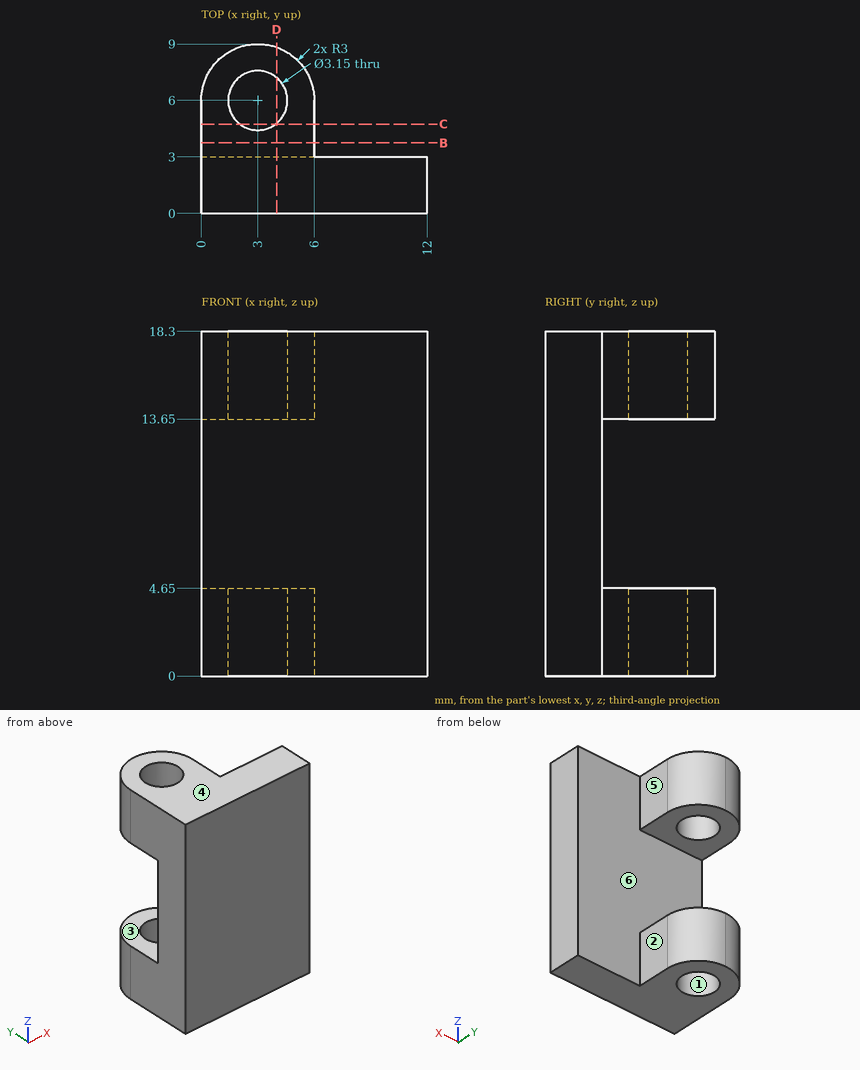
Job drawing, mm, ordinate dimensions from the low corner. One solid piece. A direction names the side the tool comes from. Round coordinates to 2 decimals unless told otherwise and drop trailing zeros. Order: outer loops, then holes, each group sorted by start corner. A loop starts at its lowest first (then second) coordinate and runs counter-clockwise, first axis right, second up. Notation, with made-up numbers: (84.25, 88) -> (138.25, 88) arc R22 cw to (138.25, 110) -> close; hole circle Ø1 at (-5.75, -17.75). An arc over 180 degrees is marked (long way). Write item = value, one per line.
(1) 3-axis set-ups, long thin cutter, end or side, ignore diameter. For the marked faces 1, 2 and 3: which of +Z, -Z, +X, -X, +Y, -Y reach the whole face in a straight line?
Answers follow:
face_1 = +Z, -Z
face_2 = +Z, -Z, +X, +Y
face_3 = +X, -X, +Y
(2) Cut at C-C (y = 4.75). Write the cut outline in (x, z).
Answers follow:
outline = (0, 0) -> (2.04, 0) -> (2.04, 4.65) -> (0, 4.65) -> close; (0, 13.65) -> (2.04, 13.65) -> (2.04, 18.3) -> (0, 18.3) -> close; (3.96, 0) -> (6, 0) -> (6, 4.65) -> (3.96, 4.65) -> close; (3.96, 13.65) -> (6, 13.65) -> (6, 18.3) -> (3.96, 18.3) -> close
(3) Cut at B-B (y = 3.75). Write the cut outline in (x, z).
Answers follow:
outline = (0, 0) -> (6, 0) -> (6, 4.65) -> (0, 4.65) -> close; (0, 13.65) -> (6, 13.65) -> (6, 18.3) -> (0, 18.3) -> close
(4) Pull direction Z, two halves, no side cores. Call the marked faces 4, 5 and 6: +Z half, -Z half, draft (parallel to the pull), parting line (faces both ways), or undercut.
Answers follow:
face_4 = +Z half
face_5 = draft
face_6 = undercut
(5) Cut at D-D (x = 4). Write the cut outline in (y, z), plus the area to 3 significant figures.
Answers follow:
outline = (0, 0) -> (4.78, 0) -> (4.78, 4.65) -> (3, 4.65) -> (3, 13.65) -> (4.78, 13.65) -> (4.78, 18.3) -> (0, 18.3) -> close; (7.22, 0) -> (8.83, 0) -> (8.83, 4.65) -> (7.22, 4.65) -> close; (7.22, 13.65) -> (8.83, 13.65) -> (8.83, 18.3) -> (7.22, 18.3) -> close
area = 86.5 mm²
(6) Drill centre lines: L1, parallel to Z at x = 4.5, y = 7.5; L2, parallel to Y at x = 3, z = 16.9 (3 decimals); L3, parallel to Y at x = 6.5, z = 15.5. Where is each one in solid material? Low to high.
Answers follow:
L1 = 0 to 4.65, 13.65 to 18.3
L2 = 0 to 4.425, 7.575 to 9
L3 = 0 to 3
(7) Flat gauge pins, fed straight in: P1, Ø2, axis at x = 9.5, z = 12, coming from the -Y side; P2, Ø1, axis at y = 8, z = 13.5, coming from the +X side (1 decimal); P3, Ø2.5, axis at y = 5, z = 17, coming from the +X side; P4, Ø5, axis at x = 9, z = 7, coming from the +Y side. Where does each tip first touch, or does it go through?
Answers follow:
P1 = 0
P2 = 5.6
P3 = 6
P4 = 3
